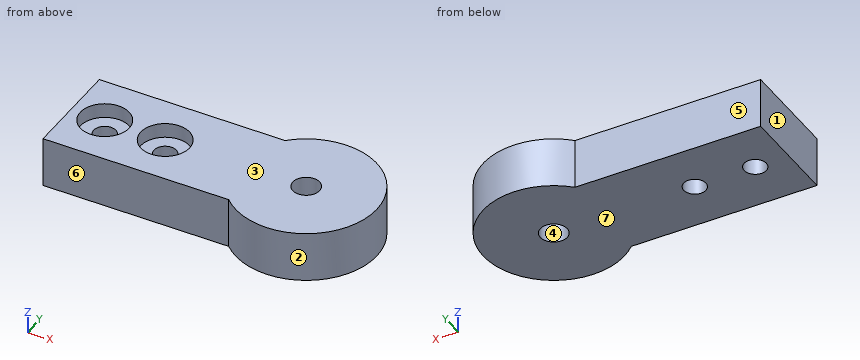
```python
from build123d import *

# Parameters (mm, degrees)
BOSS_EXTRUDE1_DEPTH                     = 15
CBORE_FOR_M6_HEX_HEAD_BOLT1_D           = 6.6
CBORE_FOR_M6_HEX_HEAD_BOLT1_CBORE_D     = 14.55
CBORE_FOR_M6_HEX_HEAD_BOLT1_CBORE_DEPTH = 4.38
CUT_EXTRUDE1_REACH                      = 76.606
SKETCH4_R                               = 4


with BuildPart() as part:
    # Sketch1 → Boss-Extrude1 (new body)
    with BuildSketch(Plane.XY):
        with BuildLine():
            Line((-14.696938457, 15), (-70, 15))
            Line((-70, 15), (-70, -15))
            Line((-70, -15), (-14.696938457, -15))
            ThreePointArc((-14.696938457, -15), (21, 0), (-14.696938457, 15))
        make_face()
    extrude(amount=BOSS_EXTRUDE1_DEPTH)

    # CBORE for M6 Hex Head Bolt1 (through all)
    with Locations(Plane.XY.offset(15)):
        with Locations((-60, 0), (-42, 0)):
            CounterBoreHole(CBORE_FOR_M6_HEX_HEAD_BOLT1_D / 2, CBORE_FOR_M6_HEX_HEAD_BOLT1_CBORE_D / 2, CBORE_FOR_M6_HEX_HEAD_BOLT1_CBORE_DEPTH)

    # Sketch4 → Cut-Extrude1 (cut, up to next)
    with BuildSketch(Plane.XY.offset(15), mode=Mode.PRIVATE) as cut_extrude1_sk1:
        Circle(SKETCH4_R)
    cut_extrude1_tool1 = extrude(cut_extrude1_sk1.sketch, amount=-CUT_EXTRUDE1_REACH, mode=Mode.PRIVATE) & part.part
    add(cut_extrude1_tool1.solids().sort_by_distance((0, 0, 15))[0], mode=Mode.SUBTRACT)


solid = part.part
```
Source: CAD feature listing. Evaluate the final solid. Frame: model axes, mm. Face numbers are marked on the shaded views. A direction names the side the tool comes from. Give positions to 0.01 mm unless a question says otherwise; leave off trailing zeros. Write each loop counter-clockwise with the first axis right and the second up, starting at its lowest first coordinate (ties: lowest second). Pieces come first, ordered by that corner, then holes.
1. Section query A-A (x = 0). Return the cut outline in (y, z).
2. Section query D-D (x = -42). Return the cut outline in (y, z) (3 decimals).
3. Pull-direction query (X, two-part tool) for the marked faces 1, 2, 3 and 4; classes: +X half, -X half, draft (parallel to the pull), parting line (faces both ways), or undercut.
4. First-contact query: pin 1 (8.5 mm diameter, centred on x = -42, y = 0, fed in from +Z); pin 2 (16 mm diameter, centred on x = -40.5, y = 2, fed in from +Z); pin 3 (3 mm diameter, centred on x = -6.5, z = 3.5, fed in from +Y); pin 4 (4.5 mm diameter, centred on x = -49, z = 8.5, fed in from -Y). Flat tips, straight axial feed; report the tip coordinate or a pass-through.
5. Section query C-C (y = 1.5). Return the cut outline in (x, z).
6. Access query for the marked faces 5, 6 and 7. Directions: +Z, -Z, +X, -X, +Y, -Y. A direction counts if a zero-diameter tool reaches every point of the face in a straight line with its end or side. Return the directions, or none.
7. Material intervals for line 1 along Y through (x, z) = (-60, 12.55) (3 decimals); line 2 along Y through (x, z) = (0, 5.75); line 3 along Y through (x, z) = (-18.5, 4.75), sorted ascending.
8. Section query B-B (z = 13). Return the cut outline in (x, y) (3 decimals), then the cut area to 3 significant figures.
Output values:
1. outline: (-21, 0) - (-4, 0) - (-4, 15) - (-21, 15) - close; (4, 0) - (21, 0) - (21, 15) - (4, 15) - close
2. outline: (-15, 0) - (-3.3, 0) - (-3.3, 10.62) - (-7.275, 10.62) - (-7.275, 15) - (-15, 15) - close; (3.3, 0) - (15, 0) - (15, 15) - (7.275, 15) - (7.275, 10.62) - (3.3, 10.62) - close
3. face 1: -X half
3. face 2: parting line
3. face 3: draft
3. face 4: undercut
4. pin 1: stops at z = 10.62
4. pin 2: stops at z = 15
4. pin 3: stops at y = 20.4
4. pin 4: stops at y = -15
5. outline: (-70, 0) - (-62.94, 0) - (-62.94, 10.62) - (-67.12, 10.62) - (-67.12, 15) - (-70, 15) - close; (-57.06, 0) - (-44.94, 0) - (-44.94, 10.62) - (-49.12, 10.62) - (-49.12, 15) - (-52.88, 15) - (-52.88, 10.62) - (-57.06, 10.62) - close; (-39.06, 0) - (-3.71, 0) - (-3.71, 15) - (-34.88, 15) - (-34.88, 10.62) - (-39.06, 10.62) - close; (3.71, 0) - (20.95, 0) - (20.95, 15) - (3.71, 15) - close
6. face 5: +Z, -Z, -X, +Y
6. face 6: +Z, -Z, -X, -Y
6. face 7: -Z, +X, -X, +Y, -Y
7. line 1: y = -15 to -7.275, 7.275 to 15
7. line 2: y = -21 to -4, 4 to 21
7. line 3: y = -15 to 15
8. outline: (-70, -15) - (-14.697, -15) arc R21 ccw (long way) to (-14.697, 15) - (-70, 15) - close; hole circle Ø14.55 at (-60, 0); hole circle Ø14.55 at (-42, 0); hole circle Ø8 at (0, 0)
8. area: 2,530 mm2
